The model under review builds one solid part; all positions refer to its coordinate system, in mm. A direction names the side the tool comes from. Give positions to 0.01 mm unless a question says otherwise; leave off trailing zeros. Loops run counter-clockwise (first coordinate to the right, second up) from the corner with the lowest first, then second, coordinate; pieces in that order, holes last. Notation, with made-up numbers: (-35, -5) - (-28, -5) arc R8 ccw to (-28, 7) - close; hole circle Ø8 at (-33.75, -11). An arc over 180 degrees is marked (long way). Answer as a JSON object with one key per item and string values.
from build123d import *

# Parameters (mm, degrees)
SKETCH1_R           = 8
BOSS_EXTRUDE1_DEPTH = 50
SKETCH2_R           = 10
BOSS_EXTRUDE2_DEPTH = 35
SKETCH3_W           = 48
SKETCH3_H           = 42
CUT_EXTRUDE1_DEPTH  = 35
SKETCH4_W           = 48
SKETCH4_H           = 0.81
CUT_EXTRUDE2_DEPTH  = 74.620649277
CUT_EXTRUDE3_REACH  = 98.322


with BuildPart() as part:
    # Sketch1 → Boss-Extrude1 (new, symmetric)
    with BuildSketch(Plane(origin=(0, 0, 0), x_dir=(0, 0, -1), z_dir=(1, 0, 0))):
        Circle(SKETCH1_R)
    extrude(amount=BOSS_EXTRUDE1_DEPTH, both=True)

    # Sketch2 → Boss-Extrude2 (add, symmetric)
    with BuildSketch(Plane(origin=(0, 0, 0), x_dir=(0, 0, -1), z_dir=(1, 0, 0))):
        with BuildLine():
            Line((-17, 25), (-17, -15))
            Line((-17, -15), (17, -15))
            Line((17, -15), (17, 25))
            ThreePointArc((17, 25), (0, 42), (-17, 25))
        make_face()
        with Locations((0, 25)):
            Circle(SKETCH2_R, mode=Mode.SUBTRACT)
    extrude(amount=BOSS_EXTRUDE2_DEPTH, both=True)

    # Sketch3 → Cut-Extrude1 (cut, symmetric)
    with BuildSketch(Plane.XY):
        with Locations((0, 21)):
            Rectangle(SKETCH3_W, SKETCH3_H)
    extrude(amount=CUT_EXTRUDE1_DEPTH, both=True, mode=Mode.SUBTRACT)

    # Sketch4 → Cut-Extrude2 (cut, through all)
    with BuildSketch(Plane(origin=(0, 0, -17), x_dir=(-1, 0, 0), z_dir=(0, 0, -1))):
        with Locations((0, -0.405)):
            Rectangle(SKETCH4_W, SKETCH4_H)
    extrude(amount=-CUT_EXTRUDE2_DEPTH, mode=Mode.SUBTRACT)

    # Cut-Extrude3: up to this face of the body (flat: up to its plane)
    cut_extrude3_end = Plane(part.part.faces().sort_by_distance((35, 10.448870599, 0))[0])
    # Sketch5 → Cut-Extrude3 (cut, up to the picked face)
    with BuildSketch(Plane.ZY.offset(35), mode=Mode.PRIVATE) as cut_extrude3_sk1:
        with BuildLine():
            Line((-7.14443883, 40.425854719), (-4.202611077, 34.074032187))
            ThreePointArc((-4.202611077, 34.074032187), (0, 35), (4.202611077, 34.074032187))
            Line((4.202611077, 34.074032187), (7.14443883, 40.425854719))
            ThreePointArc((7.14443883, 40.425854719), (0, 42), (-7.14443883, 40.425854719))
        make_face()
    cut_extrude3_tool1 = split(extrude(cut_extrude3_sk1.sketch, amount=-CUT_EXTRUDE3_REACH, mode=Mode.PRIVATE), bisect_by=cut_extrude3_end, keep=Keep.BOTH, mode=Mode.PRIVATE)
    add(cut_extrude3_tool1.solids().sort_by(Axis((-35, 38.373758, 0), (1, 0, 0)))[0], mode=Mode.SUBTRACT)


solid = part.part
Q1. Consider section D-D, the plane z = 5.5. State the section outline as (x, y) points.
Results:
{"outline": "(-50, -5.81) - (-35, -5.81) - (-35, -15) - (35, -15) - (35, -5.81) - (50, -5.81) - (50, 5.81) - (35, 5.81) - (35, 16.65) - (24, 16.65) - (24, -0.81) - (-24, -0.81) - (-24, 16.65) - (-35, 16.65) - (-35, 5.81) - (-50, 5.81) - close; (-35, 33.35) - (-24, 33.35) - (-24, 36.88) - (-35, 36.88) - close; (24, 33.35) - (35, 33.35) - (35, 36.88) - (24, 36.88) - close"}
Q2. For faces 5 (the face through (42.6, -7.81, 1.73)), 6 (the face through (-42.4, -7.81, 1.73)), 7 (the face through (29.423, 37.205, 5.653)), list the 3-axis set-ups (+Z, -Z, +X, -X, +Y, -Y) from which the entire face can be reached by the end or side of a thin tool; tool diameter is ignored.
Results:
{"face 5": "+X", "face 6": "-X", "face 7": "+X, -X, +Y"}
Q3. Consider section B-B, the plane x = 28. State the section outline as (y, z) points, plus the area to 3 significant figures.
Results:
{"outline": "(-15, -17) - (25, -17) arc R17 ccw to (40.43, -7.14) - (34.07, -4.2) arc R10 cw (long way) to (34.07, 4.2) - (40.43, 7.14) arc R17 ccw to (25, 17) - (-15, 17) - close", "area": "1,420 mm^2"}
Q4. Consider section C-C, the plane z = 0. State the section outline as (x, y) points, plus the area to 3 significant figures.
Results:
{"outline": "(-50, -8) - (-35, -8) - (-35, -15) - (35, -15) - (35, -8) - (50, -8) - (50, 8) - (35, 8) - (35, 15) - (24, 15) - (24, -0.81) - (-24, -0.81) - (-24, 15) - (-35, 15) - (-35, 8) - (-50, 8) - close", "area": "1,820 mm^2"}
Q5. Clearance check with a flat-ended pin moving along its axis: pin 1 Ø17 at (y, z) = (18, -8.5) entering from +X. State where the tip first meets the part, or that it passes through.
Results:
{"pin 1": "stops at x = 35"}
Q6. To check wall thickness, follow probe 1 along X at (y, z) = (21, 14.5); probe 2 along Z at (x, y) = (30, 25); probe 3 along X at (y, z) = (4.5, 0). State the ranges of each line that lie inside material, in increasing order. Write a range as [from, to].
Results:
{"probe 1": "x = [-35, -24], [24, 35]", "probe 2": "z = [-17, -10], [10, 17]", "probe 3": "x = [-50, -24], [24, 50]"}
Q7. Consider section A-A, the plane y = 24. State the section outline as (x, z) points, plus the area to 3 significant figures.
Results:
{"outline": "(-35, -17) - (-24, -17) - (-24, -9.95) - (-35, -9.95) - close; (-35, 9.95) - (-24, 9.95) - (-24, 17) - (-35, 17) - close; (24, -17) - (35, -17) - (35, -9.95) - (24, -9.95) - close; (24, 9.95) - (35, 9.95) - (35, 17) - (24, 17) - close", "area": "310 mm^2"}
Q8. The part is to be moulded in two halves that separate along Y. For faces 1 (the face through (-30, 15, 0)), 2 (the face through (0, -4, -17)), 3 (the face through (0, -0.81, 0)), 4 (the face through (29, 15, 0)), say which applies: +Y half, -Y half, draft (parallel to the pull), parting line (faces both ways), or undercut.
Results:
{"face 1": "undercut", "face 2": "draft", "face 3": "+Y half", "face 4": "undercut"}
